Source: CAD feature listing. Evaluate the final solid. Frame: model axes, mm. Face numbers are marked on the shaded views. A direction names the side the tool comes from. Round coordinates to 2 decimals unless told otherwise and drop trailing zeros. Write each loop counter-clockwise with the first axis right and the second up, starting at its lowest first coordinate (ties: lowest second). Pieces come first, ordered by that corner, then holes. Notation, with made-up numbers: M 86.25,22 L 108.25,22 A22 cw 108.25,60 Z; hole C -0.5,35.25 d10. An arc over 180 degrees is marked long. Answer in a Markdown table with one row per item. Add a question column.
Item 1: Cut plane D-D on z = -9.75. Return loops of the section in (x, y).
Item 2: Cut plane A-A on z = 0. Return loops of the section in (x, y), and give its area (3 significant figures).
Item 3: Set-up query: the marked faces 1, 2 and 3. Return all of +Z, -Z, +X, -X, +Y, -Y with unobstructed straight access to the full face (end or side cutting, diameter ignored); none if empty.
Item 4: Cut plane C-C on y = 8. Return loops of the section in (x, z), and give its area (3 significant figures).
Item 5: Cut plane B-B on x = 4.82. Return loops of the section in (y, z), and give its area (3 significant figures).
Item 6: Contact query for flat-ended pins moving along their axis: pin 1 (1.1 mm diameter, centred on x = 5, y = 9, fed in from -Z); pin 2 (0.8 mm diameter, centred on x = -5, y = 9.5, fed in from +Z); pin 3 (2.5 mm diameter, centred on y = 9, z = 0, fed in from -X). Output: stop coordinate, or through.
Item 7: Material intervals for probe 1 along Y at (x, z) = (-4.82, 1.95); probe 2 along Z at (x, y) = (-0.5, 9); probe 3 along Y at (x, z) = (-10.25, 1.75), sorted ascending.
from build123d import *

# Parameters (mm, degrees)
IZIM1_W                     = 23.88
IZIM1_H                     = 10.92
Y_KSEKLIK_EKSTR_ZYON5_DEPTH = 10
IZIM4_W                     = 60
IZIM4_H                     = 60
Y_KSEKLIK_EKSTR_ZYON6_DEPTH = 5
IZIM5_R                     = 1
KES_EKSTR_ZYON1_DEPTH       = 3
IZIM6_R                     = 1
KES_EKSTR_ZYON2_DEPTH       = 3
L_EK1_SCALE                 = 0.5


with BuildPart() as part:
    # Çizim1 → Yükseklik-Ekstrüzyon5 (new body)
    with BuildSketch(Plane(origin=(0, 0, 0), x_dir=(1, 0, 0), z_dir=(0, 1, 0))):
        Rectangle(IZIM1_W, IZIM1_H)
    extrude(amount=Y_KSEKLIK_EKSTR_ZYON5_DEPTH)

    # Çizim4 → Yükseklik-Ekstrüzyon6 (add)
    with BuildSketch(Plane(origin=(0, 10, 0), x_dir=(1, 0, 0), z_dir=(0, 1, 0))):
        Rectangle(IZIM4_W, IZIM4_H)
    extrude(amount=Y_KSEKLIK_EKSTR_ZYON6_DEPTH)

    # Çizim5 → Kes-Ekstrüzyon1 (cut)
    with BuildSketch(Plane.XY.offset(5.46)):
        with Locations((9.64, 2.25)):
            Circle(IZIM5_R)
        with Locations((9.64, 6.75)):
            Circle(IZIM5_R)
        with Locations((-9.64, 6.75)):
            Circle(IZIM5_R)
        with Locations((-9.64, 2.25)):
            Circle(IZIM5_R)
    extrude(amount=-KES_EKSTR_ZYON1_DEPTH, mode=Mode.SUBTRACT)

    # Çizim6 → Kes-Ekstrüzyon2 (cut)
    with BuildSketch(Plane(origin=(0, 0, -5.46), x_dir=(-1, 0, 0), z_dir=(0, 0, -1))):
        with Locations((9.64, 2.25)):
            Circle(IZIM6_R)
        with Locations((9.64, 6.75)):
            Circle(IZIM6_R)
        with Locations((-9.64, 6.75)):
            Circle(IZIM6_R)
        with Locations((-9.64, 2.25)):
            Circle(IZIM6_R)
    extrude(amount=-KES_EKSTR_ZYON2_DEPTH, mode=Mode.SUBTRACT)


with BuildPart() as part_1:
    # Ölçek1: scaled about (0, 11.57684301, 0)
    add(part.part.scale(L_EK1_SCALE).moved(Location((0, 5.788421505, 0))))


solid = part_1.part
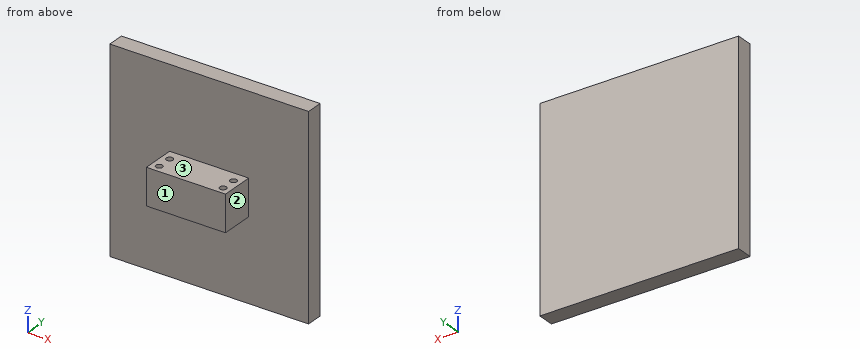
Results below:
| question | item | result |
|---|---|---|
| 1 | outline | M -15,10.79 L 15,10.79 L 15,13.29 L -15,13.29 Z |
| 2 | outline | M -15,10.79 L -5.97,10.79 L -5.97,5.79 L 5.97,5.79 L 5.97,10.79 L 15,10.79 L 15,13.29 L -15,13.29 Z |
| 2 | area | 135 mm2 |
| 3 | face 1 | +Z, -Z, +X, -X, -Y |
| 3 | face 2 | +Z, -Z, +X, -Y |
| 3 | face 3 | +Z, +X, -X, -Y |
| 4 | outline | M -5.97,-2.73 L 5.97,-2.73 L 5.97,2.73 L -5.97,2.73 Z |
| 4 | area | 65.2 mm2 |
| 5 | outline | M 5.79,-2.73 L 6.41,-2.73 L 6.41,-1.23 L 7.41,-1.23 L 7.41,-2.73 L 8.66,-2.73 L 8.66,-1.23 L 9.66,-1.23 L 9.66,-2.73 L 10.79,-2.73 L 10.79,-15 L 13.29,-15 L 13.29,15 L 10.79,15 L 10.79,2.73 L 9.66,2.73 L 9.66,1.23 L 8.66,1.23 L 8.66,2.73 L 7.41,2.73 L 7.41,1.23 L 6.41,1.23 L 6.41,2.73 L 5.79,2.73 Z |
| 5 | area | 96.3 mm2 |
| 6 | pin 1 | z = -2.73 |
| 6 | pin 2 | z = 2.73 |
| 6 | pin 3 | x = -5.97 |
| 7 | probe 1 | 5.79 to 6.41, 7.41 to 8.66, 9.66 to 13.29 |
| 7 | probe 2 | -2.73 to 2.73 |
| 7 | probe 3 | 10.79 to 13.29 |
